Part model, mm, in its own coordinate system. A direction names the side the tool comes from. Give positions to 0.01 mm unless a question says otherwise; leave off trailing zeros. Order: outer loops, then holes, each group sorted by start corner. A loop starts at its lowest first (then second) coordinate and runs counter-clockwise, first axis right, second up. Notation, with made-up numbers: (39.5, 18.5) - (93.5, 18.5) arc R23 cw to (93.5, 47.5) - close; hole circle Ø5 at (58.5, 44). An arc over 180 degrees is marked (long way). One line per item, written item: value.
```python
from build123d import *

# Parameters (mm, degrees)
SKETCH4_W           = 29
SKETCH4_H           = 59
BOSS_EXTRUDE2_DEPTH = 43
SKETCH5_W           = 29
SKETCH5_H           = 74
BOSS_EXTRUDE3_DEPTH = 4
SKETCH6_W           = 29
SKETCH6_H           = 59
BOSS_EXTRUDE4_DEPTH = 2
SKETCH7_W           = 27
SKETCH7_H           = 57
BOSS_EXTRUDE5_DEPTH = 1
SKETCH8_W           = 27
SKETCH8_H           = 47
BOSS_EXTRUDE7_DEPTH = 3.99
SKETCH11_R          = 7
BOSS_EXTRUDE8_DEPTH = 3
SKETCH12_R          = 3
BOSS_EXTRUDE9_DEPTH = 4
SKETCH13_R          = 2.5
CUT_EXTRUDE1_DEPTH  = 4


with BuildPart() as part:
    # Sketch4 → Boss-Extrude2 (new body)
    with BuildSketch(Plane.XY):
        with Locations((-44.629997068, -10.100928214)):
            Rectangle(SKETCH4_W, SKETCH4_H)
    extrude(amount=BOSS_EXTRUDE2_DEPTH)

    # Sketch5 → Boss-Extrude3 (add)
    with BuildSketch(Plane.XY.offset(43)):
        with Locations((-44.629997068, -10.100928214)):
            Rectangle(SKETCH5_W, SKETCH5_H)
    extrude(amount=-BOSS_EXTRUDE3_DEPTH)

    # Sketch6 → Boss-Extrude4 (add)
    with BuildSketch(Plane.XY.offset(43)):
        with Locations((-44.629997068, -10.100928214)):
            Rectangle(SKETCH6_W, SKETCH6_H)
    extrude(amount=BOSS_EXTRUDE4_DEPTH)

    # Sketch7 → Boss-Extrude5 (add)
    with BuildSketch(Plane.XY.offset(45)):
        with Locations((-44.629997068, -10.100928214)):
            Rectangle(SKETCH7_W, SKETCH7_H)
    extrude(amount=BOSS_EXTRUDE5_DEPTH)

    # Sketch8 → Boss-Extrude7 (add)
    with BuildSketch(Plane.XY.offset(46)):
        with Locations((-44.629997068, -4.100928214)):
            Rectangle(SKETCH8_W, SKETCH8_H)
    extrude(amount=BOSS_EXTRUDE7_DEPTH)

    # Sketch11 → Boss-Extrude8 (add)
    with BuildSketch(Plane.XY.offset(49.99)):
        with Locations((-45.129997068, 5.399071786)):
            Circle(SKETCH11_R)
    extrude(amount=BOSS_EXTRUDE8_DEPTH)

    # Sketch12 → Boss-Extrude9 (add)
    with BuildSketch(Plane.XY.offset(52.99)):
        with Locations((-45.129997068, 5.399071786)):
            Circle(SKETCH12_R)
    extrude(amount=BOSS_EXTRUDE9_DEPTH)

    # Sketch13 → Cut-Extrude1 (cut)
    with BuildSketch(Plane.XY.offset(43)):
        with Locations((-36.629997068, 23.899071786)):
            Circle(SKETCH13_R)
        with Locations((-52.629997068, 23.899071786)):
            Circle(SKETCH13_R)
        with Locations((-52.629997068, -44.100928214)):
            Circle(SKETCH13_R)
        with Locations((-36.629997068, -44.100928214)):
            Circle(SKETCH13_R)
    extrude(amount=-CUT_EXTRUDE1_DEPTH, mode=Mode.SUBTRACT)


solid = part.part
```
1) Wall check: line 1 along Z through (x, y) = (-55.75, 6); line 2 along Y through (x, z) = (-44, 13); line 3 along X through (y, z) = (12, 49.5). Give the ranges that are in metal, low to high. Write a range as [from, to].
Answer:
line 1: z = [0, 49.99]
line 2: y = [-39.6, 19.4]
line 3: x = [-58.13, -31.13]
2) Two-plate mould, pull along Y, no slides. Class faces 6 (the face through (-45, -4, 49.99)), 7 (the face through (-39.128, 24.009, 41.028)), 8 (the face through (-45, -39.601, 44)): pulls with the +Y half, pulls with the -Y half, needs draft (parallel to the pull), parting line crosses it, or undercut.
Answer:
face 6: needs draft
face 7: undercut
face 8: pulls with the -Y half
3) Slice it at A-A on y = -37. Write the cut outline in (x, z), then the cut area to 3 significant figures.
Answer:
outline: (-59.13, 0) - (-30.13, 0) - (-30.13, 45) - (-31.13, 45) - (-31.13, 46) - (-58.13, 46) - (-58.13, 45) - (-59.13, 45) - close
area: 1,330 mm2
4) Slice it at C-C on z = 47.5. Write the cut outline in (x, y), then the cut area to 3 significant figures.
Answer:
outline: (-58.13, -27.6) - (-31.13, -27.6) - (-31.13, 19.4) - (-58.13, 19.4) - close
area: 1,270 mm2
5) Slice it at D-D on y = -11.5. Write the cut outline in (x, z).
Answer:
outline: (-59.13, 0) - (-30.13, 0) - (-30.13, 45) - (-31.13, 45) - (-31.13, 49.99) - (-58.13, 49.99) - (-58.13, 45) - (-59.13, 45) - close
6) Drop flat-ended pins along their axis: P1, Ø2, axis at x = -50, y = 23, coming from the -Z side; P2, Ø14.5, axis at x = -41, z = 18, coming from the +Y side; P3, Ø2.5, axis at y = -4.5, z = 48.5, coming from the +X side. Give the stop position or say it passes through.
Answer:
P1: stops at z = 39
P2: stops at y = 19.4
P3: stops at x = -31.13
7) Slice it at B-B on x = -54.25. Write the cut outline in (y, z), then the cut area to 3 significant figures.
Answer:
outline: (-47.1, 39) - (-46.01, 39) - (-46.01, 43) - (-47.1, 43) - close; (-42.2, 39) - (-39.6, 39) - (-39.6, 0) - (19.4, 0) - (19.4, 39) - (21.99, 39) - (21.99, 43) - (19.4, 43) - (19.4, 45) - (18.4, 45) - (18.4, 46) - (19.4, 46) - (19.4, 49.99) - (-27.6, 49.99) - (-27.6, 46) - (-38.6, 46) - (-38.6, 45) - (-39.6, 45) - (-39.6, 43) - (-42.2, 43) - close; (25.8, 39) - (26.9, 39) - (26.9, 43) - (25.8, 43) - close
area: 2,930 mm2
8) Which spindle directions (+Z, -Z, +X, -X, +Y, -Y) get a long thin tool onto all of the face, cutting with end or side? Do faces 1 (the face through (-45, -39.601, 19)), 2 (the face through (-31.13, -4, 47)), 3 (the face through (-45, 19.399, 44)), 4 (the face through (-45, 19.399, 19)), 5 (the face through (-45, -43, 43)). Say none if no direction does.
Answer:
face 1: -Z, +X, -X, -Y
face 2: +Z, +X, +Y, -Y
face 3: +Z, +X, -X, +Y
face 4: -Z, +X, -X, +Y
face 5: +Z, +X, -X, -Y
